Job drawing, mm, ordinate dimensions from the low corner. One solid piece. Give positions to 0.01 mm unless a question says otherwise; leave off trailing zeros. Write each loop counter-clockwise with the first axis right and the second up, starting at its lowest first coordinate (ties: lowest second). Pieces come first, ordered by that corner, then holes. Notation, with made-up numbers: (42.25, 35.5) - (68.25, 35.5) arc R33 cw to (68.25, 67.5) - close; hole circle Ø8 at (13, 54.5). An arc over 180 degrees is marked (long way). Answer as a JSON object with one key per item and string values.
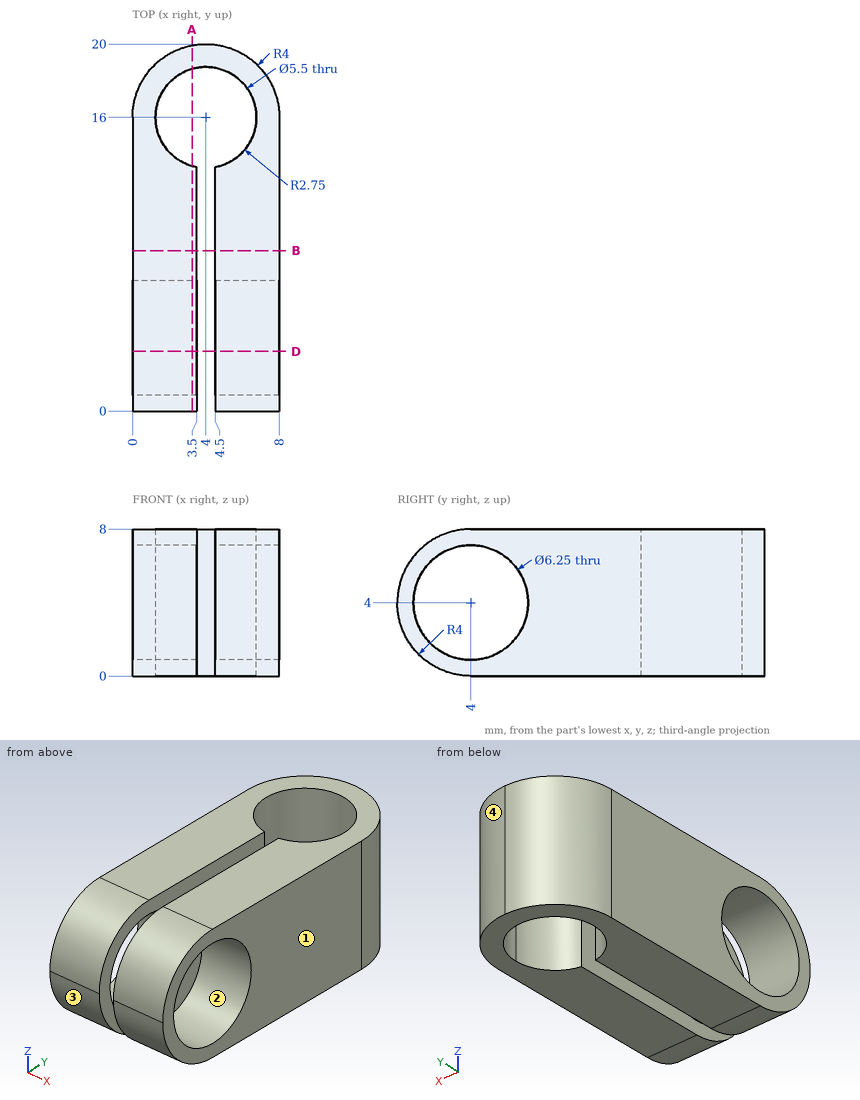
Item 1: Cut at B-B (y = 8.75). Give the cut face in (x, z), and give its area (3 significant figures).
Entries:
{"outline": "(0, 0) - (3.5, 0) - (3.5, 8) - (0, 8) - close; (4.5, 0) - (8, 0) - (8, 8) - (4.5, 8) - close", "area": "56.0 mm2"}
Item 2: Cut at D-D (y = 3.25). Give the cut face in (x, z).
Entries:
{"outline": "(0, 0.07) - (3.5, 0.07) - (3.5, 0.97) - (0, 0.97) - close; (0, 7.03) - (3.5, 7.03) - (3.5, 7.93) - (0, 7.93) - close; (4.5, 0.07) - (8, 0.07) - (8, 0.97) - (4.5, 0.97) - close; (4.5, 7.03) - (8, 7.03) - (8, 7.93) - (4.5, 7.93) - close"}
Item 3: Cut at A-A (x = 3.25). State how many separate pieces and enclosed holes the cut face has, and give its area (3 significant figures).
Entries:
{"separate pieces": "2", "enclosed holes": "1", "area": "79.6 mm2"}
Item 4: Mould opens along Y. For the marked faces 1, 2, 3 and 4 say: +Y half, -Y half, draft (parallel to the pull), parting line (faces both ways), or undercut.
Entries:
{"face 1": "draft", "face 2": "undercut", "face 3": "-Y half", "face 4": "+Y half"}
Item 5: Probe line 1 (Z direction, x = 6.55, y = 4) (3 decimals); line 2 (X direction, y = 3.75, z = 7.25); line 3 (Y direction, x = 5.65, z = 4) (3 decimals). List the from-to ranges inside material, lowest first. Write a range as from..to.
Entries:
{"line 1": "0..0.875, 7.125..8", "line 2": "0..3.5, 4.5..8", "line 3": "0..0.875, 7.125..13.8, 18.2..19.644"}
